Input: part model. Units: mm. Frame: model coordinates. Coordinates: 2 decimals unless noted, no trailing zeros. Order: outer loops, then holes, each group sorted by start corner. A loop starts at its lowest first (then second) coordinate and runs counter-clockwise, first axis right, second up. Notation, with made-up numbers: M -32,19.25 L -22,19.25 A14 cw -22,37.25 Z; hole C 89.25,44 d9. An arc over 180 degrees is marked long. One line per item, written item: value.
```python
from build123d import *

# Parameters (mm, degrees)
REVOLVE_1_ANGLE           = 98.68117871
REVOLVE_1_OTHER_WAY_ANGLE = 8.68117871
SKETCH_3_R                = 4
CUT_EXTRUDE_1_DEPTH       = 94.680307429
SKETCH_4_R                = 4
CUT_EXTRUDE_2_DEPTH       = 94.59487173
FILLET_START              = -16.507933569
FILLET_1_DEPTH            = 83.507933569
FILLET_START_2            = -67
FILLET_1_2_DEPTH          = 83.255659247


with BuildPart() as part:
    # 草图2 → 旋转1 (revolve)
    with BuildSketch(Plane.XY):
        with BuildLine():
            Line((61.481704596, 8), (65.513357417, 8))
            ThreePointArc((65.513357417, 8), (66, 0), (65.513357417, -8))
            Line((65.513357417, -8), (61.481704596, -8))
            ThreePointArc((61.481704596, -8), (62, 0), (61.481704596, 8))
        make_face()
    revolve(axis=Axis((0, 0, 0), (0, -1, 0)), revolution_arc=REVOLVE_1_ANGLE)

    # 草图2 → 旋转1 other way (revolve)
    with BuildSketch(Plane.XY):
        with BuildLine():
            Line((61.481704596, 8), (65.513357417, 8))
            ThreePointArc((65.513357417, 8), (66, 0), (65.513357417, -8))
            Line((65.513357417, -8), (61.481704596, -8))
            ThreePointArc((61.481704596, -8), (62, 0), (61.481704596, 8))
        make_face()
    revolve(axis=Axis((0, 0, 0), (0, 1, 0)), revolution_arc=REVOLVE_1_OTHER_WAY_ANGLE)

    # 草图3 → 切除-拉伸1 (cut, through all)
    with BuildSketch(Plane.XY):
        with Locations(Location((0, 0, 0), (0, 0, 180))):
            Circle(SKETCH_3_R)
    extrude(amount=CUT_EXTRUDE_1_DEPTH, mode=Mode.SUBTRACT)

    # 草图4 → 切除-拉伸2 (cut, through all)
    with BuildSketch(Plane(origin=(0, 0, 0), x_dir=(0, 0, -1), z_dir=(1, 0, 0))):
        with Locations(Location((0, 0, 0), (0, 0, 180))):
            Circle(SKETCH_4_R)
    extrude(amount=CUT_EXTRUDE_2_DEPTH, mode=Mode.SUBTRACT)

    # 圆角1: read off the stored shape, not the designer's step
    # 圆角1 outline → 圆角1 (cut)
    with BuildSketch(Plane(origin=(0, 0, 0), x_dir=(0, 1, 0), z_dir=(0.9885435216678343, 0, -0.15093609829512605)).offset(FILLET_START)):
        with BuildLine():
            Line((8, 0), (8, 8))
            ThreePointArc((8, 8), (5.656854249, 2.343145751), (0, 0))
            Line((0, 0), (8, 0))
        make_face()
        with BuildLine():
            Line((-8, 0), (0, 0))
            ThreePointArc((0, 0), (-5.656854249, 2.343145751), (-8, 8))
            Line((-8, 8), (-8, 0))
        make_face()
    extrude(amount=FILLET_1_DEPTH, mode=Mode.SUBTRACT)

    # Fillet 1 2 outline → Fillet 1 2 (cut)
    with BuildSketch(Plane(origin=(0, 0, 0), x_dir=(0.9885435216678338, 0, 0.15093609829512997), z_dir=(0.15093609829512997, 0, -0.9885435216678338)).offset(FILLET_START_2)):
        with BuildLine():
            Line((0, -8), (8, -8))
            ThreePointArc((8, -8), (2.343145751, -5.656854249), (0, 0))
            Line((0, 0), (0, -8))
        make_face()
        with BuildLine():
            Line((0, 8), (0, 0))
            ThreePointArc((0, 0), (2.343145751, 5.656854249), (8, 8))
            Line((8, 8), (0, 8))
        make_face()
    extrude(amount=FILLET_1_2_DEPTH, mode=Mode.SUBTRACT)


solid = part.part
```
(1) Cut plane A-A on y = -3. Output: boundary loops of the cut face in (x, z).
Data:
outline: M -9.37,65.26 L -8.77,61.3 A61.93 cw -2.65,61.87 L -2.65,65.88 A65.93 ccw Z; M 2.65,61.87 A61.93 cw 61.87,2.65 L 65.88,2.65 A65.93 ccw 2.65,65.88 Z; M 61.3,-8.77 L 65.26,-9.37 A65.93 ccw 65.88,-2.65 L 61.87,-2.65 A61.93 cw Z
(2) Cut plane B-B on x = 2. Output: boundary loops of the cut face in (y, z), plus the area to 3 significant figures.
Data:
outline: M -8,61.45 A61.97 cw -3.46,61.87 L -3.46,65.88 A65.97 ccw -8,65.48 Z; M 3.46,61.87 A61.97 cw 8,61.45 L 8,65.48 A65.97 ccw 3.46,65.88 Z
area: 36.5 mm2
(3) Ray query, line 1 (Y direction, x = 62.7, z = 0); line 2 (X direction, y = 3.25, z = 53.5); line 3 (Z direction, x = 31, y = 5). Return the intervals inside material, ascending. Write a range as from..to.
Data:
line 1: y = -8..-4, 4..8
line 2: x = 31.16..38.51
line 3: z = 53.46..58.05
(4) Draft query along Y for faces 1 (the flat face through (44, -8, 44)), 2 (the cylindrical face through (63.847, 3.905, -0.867)), 3 (the flat face through (44, 8, 44)). Return one class per face: released by +Y, released by -Y, zero draft, split by the parting line, or undercut.
Data:
face 1: released by -Y
face 2: undercut
face 3: released by +Y
(5) First-contact query: pin 1 (1 mm diameter, centred on x = 28.5, y = 6, fed in from +Z); pin 2 (5 mm diameter, centred on x = 47.5, y = 0.5, fed in from +Z); pin 3 (1 mm diameter, centred on y = -3.5, z = 52, fed in from +X). Flat tips, straight axial feed; report the tip coordinate or a pass-through.
Data:
pin 1: stops at z = 59.47
pin 2: stops at z = 48.28
pin 3: stops at x = 41.13
(6) Cut plane C-C on z = 0. Output: boundary loops of the cut face in (x, y).
Data:
outline: M 61.48,-8 L 65.51,-8 A66 ccw 65.88,-4 L 61.87,-4 A62 cw Z; M 61.48,8 A62 cw 61.87,4 L 65.88,4 A66 ccw 65.51,8 Z
(7) Cut plane D-D on z = 24.5. Output: boundary loops of the cut face in (x, y).
Data:
outline: M 56.39,-8 L 60.76,-8 A61.28 ccw 60.76,8 L 56.39,8 A56.95 cw Z
